Geometry check sheet. Reference: drawing and pictorial views, mm from the part's lowest x, y, z. A direction names the side the tool comes from. Give positions to 0.01 mm unless a question says otherwise; leave off trailing zeros. Order: outer loops, then holes, each group sorted by start corner. A loop starts at its lowest first (then second) coordinate and runs counter-clockwise, first axis right, second up.
Item 1: Sectioned sample at C-C on z = 86.5. Record the boundary of the cut face in (x, y) (3 decimals).
Item 2: Material ranges on line 1 along Z through (x, y) = (63.5, 43) (3 decimals); line 2 along Z through (x, y) = (126, 72) (3 decimals); line 3 along X through (y, z) = (54.5, 95), recorded low to high.
Item 3: Access from +Z, -Z, +X, -X, +Y, -Y to the whole of each face (thin tool, end or side, straight path). Record for the marked faces 5, 6 and 7.
Item 4: Gauge pin test, flat ends, axial feed: P1, Ø4, axis at x = 154, y = 22.5, coming from the +Z side; P2, Ø12.5, axis at y = 17, z = 143, coming from the +X side; P3, Ø6, axis at x = 178.5, z = 40.5, coming from the +Y side (3 decimals). Record the tip position at first contact, or that the pin passes through.
Item 5: Release check for a two-part mould opening along X. For the marked faces 1, 2, 3 and 4 record: released by +X, released by -X, zero draft, split by the parting line, or undercut.
Item 6: Sectioned sample at B-B on y = 8.5. Record the boundary of the cut face in (x, z) (3 decimals).
Item 7: Sectioned sample at A-A on x = 190.5. Record the boundary of the cut face in (y, z) (3 decimals), and give its area (3 significant figures).
Item 8: Sectioned sample at D-D on x = 63.5. Record the boundary of the cut face in (y, z) (3 decimals).
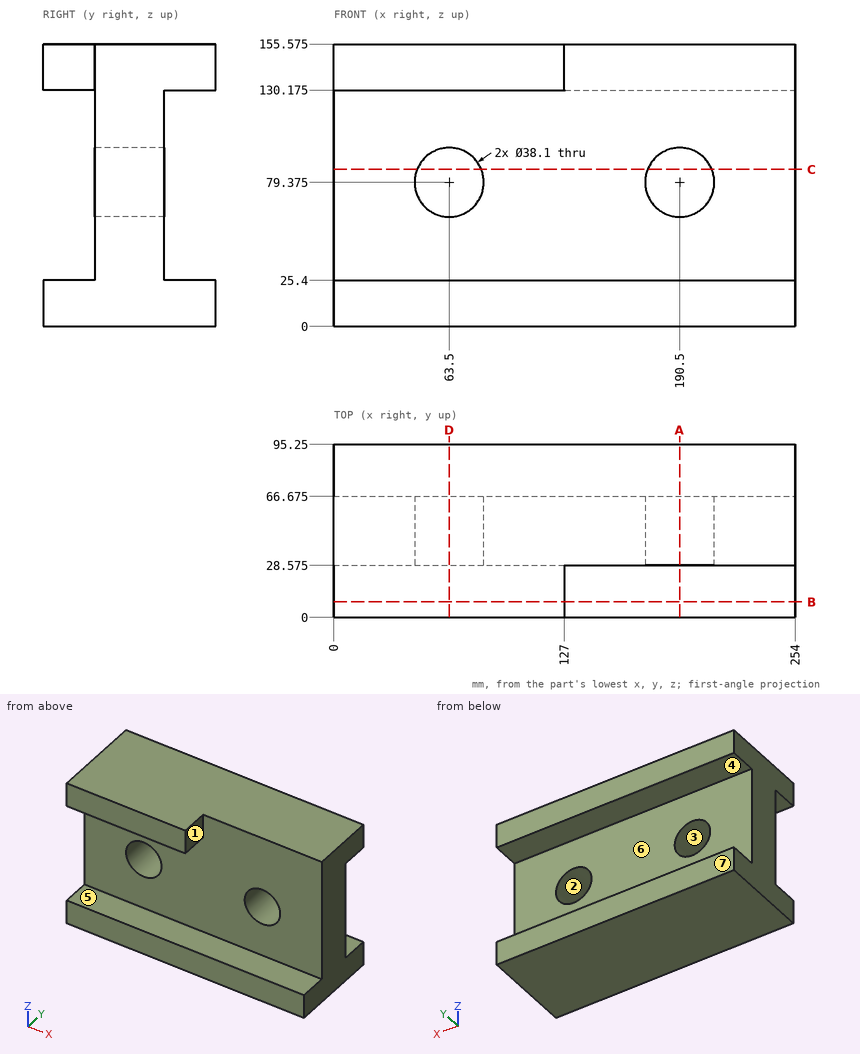
Report:
1. outline: (0, 28.575) - (45.833, 28.575) - (45.833, 66.675) - (0, 66.675) - close; (81.167, 28.575) - (172.833, 28.575) - (172.833, 66.675) - (81.167, 66.675) - close; (208.167, 28.575) - (254, 28.575) - (254, 66.675) - (208.167, 66.675) - close
2. line 1: z = 0 to 60.325, 98.425 to 155.575
2. line 2: z = 0 to 25.4, 130.175 to 155.575
2. line 3: x = 0 to 52.6, 74.4 to 179.6, 201.4 to 254
3. face 5: +X, -X, -Y
3. face 6: +X, -X, +Y
3. face 7: +Z, -Z, +X, -X, +Y
4. P1: stops at z = 25.4
4. P2: stops at x = 127
4. P3: stops at y = 66.675
5. face 1: released by +X
5. face 2: undercut
5. face 3: undercut
5. face 4: zero draft
6. outline: (0, 0) - (254, 0) - (254, 25.4) - (0, 25.4) - close; (0, 130.175) - (127, 130.175) - (127, 155.575) - (0, 155.575) - close
7. outline: (0, 0) - (95.25, 0) - (95.25, 25.4) - (66.675, 25.4) - (66.675, 60.325) - (28.575, 60.325) - (28.575, 25.4) - (0, 25.4) - close; (28.575, 98.425) - (66.675, 98.425) - (66.675, 130.175) - (95.25, 130.175) - (95.25, 155.575) - (28.575, 155.575) - close
7. area: 6,650 mm2
8. outline: (0, 0) - (95.25, 0) - (95.25, 25.4) - (66.675, 25.4) - (66.675, 60.325) - (28.575, 60.325) - (28.575, 25.4) - (0, 25.4) - close; (0, 130.175) - (28.575, 130.175) - (28.575, 98.425) - (66.675, 98.425) - (66.675, 130.175) - (95.25, 130.175) - (95.25, 155.575) - (0, 155.575) - close
